Read the model definition and answer for the solid it produces. Units are mm, in the model's axes. Face numbers are marked on the shaded views. Coordinates: 2 decimals unless noted, no trailing zeros. Write each loop counter-clockwise with the first axis right and the second up, starting at its lowest first coordinate (ties: lowest second). Pieces come first, ordered by that corner, then holes.
1) Determine the mould class of the marked faces 1, 2, 3 and 4 for opening direction X: +X half, -X half, draft (parallel to the pull), parting line (faces both ways), or undercut.
2) The part is cut by section B-B (z = 18). Determine the outline of the cut face in (x, y), then the cut area to 3 significant figures.
3) The part is cut by section C-C (y = 41). Determine the outline of the cut face in (x, z).
4) Each of these flat-tipped pins is pushed along its axis until it touches: pin 1 Ø2 at (y, z) = (11, 11) entering from +X; pin 2 Ø1.2 at (x, z) = (-2, 14) entering from -Y; pin 3 Ø12 at (x, y) = (-141.5, 29) entering from +Z; pin 4 Ø3 at (x, z) = (-1.5, 14) entering from +Y. Where does it stop, or does it pass through?
5) Find the intervals of material crossed by line 1 (Y direction, x = -169, z = 18); line 2 (X direction, y = 5, z = 25); line 3 (Z direction, x = -145, y = 23), in increasing order.
6) The part is cut by section D-D (x = -58.5). Determine the outline of the cut face in (y, z), then the cut area to 3 significant figures.
7) The part is cut by section A-A (z = 28.5). Determine the outline of the cut face in (x, y).
from build123d import *

# Parameters (mm, degrees)
CROQUIS1_W              = 171.8
CROQUIS1_H              = 48
SALIENTE_EXTRUIR1_DEPTH = 3
CROQUIS2_W              = 4
CROQUIS2_H              = 44
SALIENTE_EXTRUIR2_DEPTH = 30
CORTAR_EXTRUIR1_START   = -171.8
CROQUIS3_W              = 30
CROQUIS3_H              = 28.304126214
CORTAR_EXTRUIR1_DEPTH   = 171.8
CORTAR_EXTRUIR2_START   = -171.8
CROQUIS4_R              = 1.5
CORTAR_EXTRUIR2_DEPTH   = 171.8


with BuildPart() as part:
    # Croquis1 → Saliente-Extruir1 (new body)
    with BuildSketch(Plane.XY):
        with Locations((-85.9, 24)):
            Rectangle(CROQUIS1_W, CROQUIS1_H)
    extrude(amount=SALIENTE_EXTRUIR1_DEPTH)

    # Croquis2 → Saliente-Extruir2 (add)
    with BuildSketch(Plane.XY.offset(3)):
        with Locations((-169.8, 26)):
            Rectangle(CROQUIS2_W, CROQUIS2_H)
        with Locations((-2, 26)):
            Rectangle(CROQUIS2_W, CROQUIS2_H)
    extrude(amount=SALIENTE_EXTRUIR2_DEPTH)

    # Croquis3 → Cortar-Extruir1 (cut)
    with BuildSketch(Plane.ZY.offset(171.8).offset(CORTAR_EXTRUIR1_START)):
        with Locations((18, 33.847936893)):
            Rectangle(CROQUIS3_W, CROQUIS3_H)
    extrude(amount=CORTAR_EXTRUIR1_DEPTH, mode=Mode.SUBTRACT)

    # Croquis4 → Cortar-Extruir2 (cut)
    with BuildSketch(Plane.ZY.offset(171.8).offset(CORTAR_EXTRUIR2_START)):
        with Locations((18, 11.847936893)):
            Circle(CROQUIS4_R)
    extrude(amount=CORTAR_EXTRUIR2_DEPTH, mode=Mode.SUBTRACT)


solid = part.part
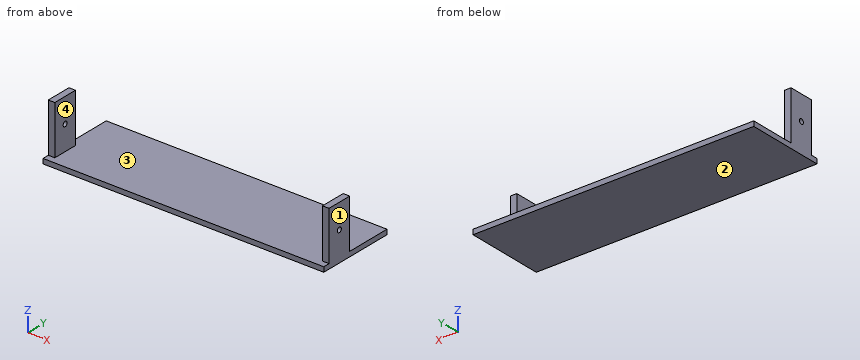
Reported:
1. face 1: +X half
1. face 2: draft
1. face 3: undercut
1. face 4: undercut
2. outline: (-171.8, 4) - (-167.8, 4) - (-167.8, 10.35) - (-171.8, 10.35) - close; (-171.8, 13.35) - (-167.8, 13.35) - (-167.8, 19.7) - (-171.8, 19.7) - close; (-4, 4) - (0, 4) - (0, 10.35) - (-4, 10.35) - close; (-4, 13.35) - (0, 13.35) - (0, 19.7) - (-4, 19.7) - close
2. area: 102 mm2
3. outline: (-171.8, 0) - (0, 0) - (0, 3) - (-171.8, 3) - close
4. pin 1: stops at x = 0
4. pin 2: stops at y = 4
4. pin 3: stops at z = 3
4. pin 4: stops at y = 19.7
5. line 1: y = 4 to 10.35, 13.35 to 19.7
5. line 2: x = -171.8 to -167.8, -4 to 0
5. line 3: z = 0 to 3
6. outline: (0, 0) - (48, 0) - (48, 3) - (0, 3) - close
6. area: 144 mm2
7. outline: (-171.8, 4) - (-167.8, 4) - (-167.8, 19.7) - (-171.8, 19.7) - close; (-4, 4) - (0, 4) - (0, 19.7) - (-4, 19.7) - close
